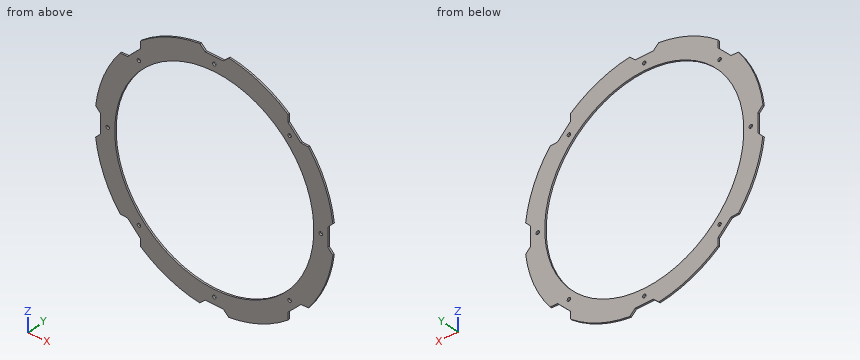
```python
from build123d import *

# Parameters (mm, degrees)
SKETCH1_R           = 3.302
SKETCH1_R_2         = 190.5
BOSS_EXTRUDE1_DEPTH = 3.175
CHAMFER1_DEPTH      = 3.175


with BuildPart() as part:
    # Sketch1 → Boss-Extrude1 (new body)
    with BuildSketch(Plane(origin=(0, 0, 0), x_dir=(1, 0, 0), z_dir=(0, 1, 0))):
        with BuildLine():
            Line((228.003026076, -16.51), (217.17, -16.51))
            Line((217.17, -16.51), (217.17, 16.51))
            Line((217.17, 16.51), (228.003026076, 16.51))
            ThreePointArc((228.003026076, 16.51), (211.198861132, 87.481432639), (172.896818827, 149.548152912))
            Line((172.896818827, 149.548152912), (165.236712628, 141.888046713))
            Line((165.236712628, 141.888046713), (141.888046713, 165.236712628))
            Line((141.888046713, 165.236712628), (149.548152912, 172.896818827))
            ThreePointArc((149.548152912, 172.896818827), (87.481432639, 211.198861132), (16.51, 228.003026076))
            Line((16.51, 228.003026076), (16.51, 217.17))
            Line((16.51, 217.17), (-16.51, 217.17))
            Line((-16.51, 217.17), (-16.51, 228.003026076))
            ThreePointArc((-16.51, 228.003026076), (-87.481432639, 211.198861132), (-149.548152912, 172.896818827))
            Line((-149.548152912, 172.896818827), (-141.888046713, 165.236712628))
            Line((-141.888046713, 165.236712628), (-165.236712628, 141.888046713))
            Line((-165.236712628, 141.888046713), (-172.896818827, 149.548152912))
            ThreePointArc((-172.896818827, 149.548152912), (-211.198861132, 87.481432639), (-228.003026076, 16.51))
            Line((-228.003026076, 16.51), (-217.17, 16.51))
            Line((-217.17, 16.51), (-217.17, -16.51))
            Line((-217.17, -16.51), (-228.003026076, -16.51))
            ThreePointArc((-228.003026076, -16.51), (-211.198861132, -87.481432639), (-172.896818827, -149.548152912))
            Line((-172.896818827, -149.548152912), (-165.236712628, -141.888046713))
            Line((-165.236712628, -141.888046713), (-141.888046713, -165.236712628))
            Line((-141.888046713, -165.236712628), (-149.548152912, -172.896818827))
            ThreePointArc((-149.548152912, -172.896818827), (-87.481432639, -211.198861132), (-16.51, -228.003026076))
            Line((-16.51, -228.003026076), (-16.51, -217.17))
            Line((-16.51, -217.17), (16.51, -217.17))
            Line((16.51, -217.17), (16.51, -228.003026076))
            ThreePointArc((16.51, -228.003026076), (87.481432639, -211.198861132), (149.548152912, -172.896818827))
            Line((149.548152912, -172.896818827), (141.888046713, -165.236712628))
            Line((141.888046713, -165.236712628), (165.236712628, -141.888046713))
            Line((165.236712628, -141.888046713), (172.896818827, -149.548152912))
            ThreePointArc((172.896818827, -149.548152912), (211.198861132, -87.481432639), (228.003026076, -16.51))
        make_face()
        with Locations(Location((-144.133110743, -144.133110743, 0), (0, 0, 270))):
            Circle(SKETCH1_R, mode=Mode.SUBTRACT)
        with Locations(Location((0, -203.835, 0), (0, 0, 270))):
            Circle(SKETCH1_R, mode=Mode.SUBTRACT)
        with Locations(Location((144.133110743, -144.133110743, 0), (0, 0, 270))):
            Circle(SKETCH1_R, mode=Mode.SUBTRACT)
        with Locations(Location((203.835, 0, 0), (0, 0, 270))):
            Circle(SKETCH1_R, mode=Mode.SUBTRACT)
        with Locations(Location((-203.835, 0, 0), (0, 0, 270))):
            Circle(SKETCH1_R, mode=Mode.SUBTRACT)
        with Locations(Location((-144.133110743, 144.133110743, 0), (0, 0, 270))):
            Circle(SKETCH1_R, mode=Mode.SUBTRACT)
        with Locations(Location((0, 0, 0), (0, 0, 270))):
            Circle(SKETCH1_R_2, mode=Mode.SUBTRACT)
        with Locations(Location((0, 203.835, 0), (0, 0, 270))):
            Circle(SKETCH1_R, mode=Mode.SUBTRACT)
        with Locations(Location((144.133110743, 144.133110743, 0), (0, 0, 270))):
            Circle(SKETCH1_R, mode=Mode.SUBTRACT)
    extrude(amount=BOSS_EXTRUDE1_DEPTH)

    # Chamfer1: read off the stored shape, not the designer's step
    # Chamfer1 outline → Chamfer1 (cut)
    with BuildSketch(Plane(origin=(0, 0, 0), x_dir=(1, 0, 0), z_dir=(0, 1, 0))):
        with BuildLine():
            ThreePointArc((228.003026076, 16.51), (227.528537531, 22.1071167), (226.916669439, 27.690885335))
            Line((226.916669439, 27.690885335), (217.17, 17.417305498))
            Line((217.17, 17.417305498), (217.17, 16.51))
            Line((217.17, 16.51), (228.003026076, 16.51))
        make_face()
        with BuildLine():
            Line((165.878274498, 141.246484842), (180.034728522, 140.873902927))
            ThreePointArc((180.034728522, 140.873902927), (176.519063933, 145.254879671), (172.896818827, 149.548152912))
            Line((172.896818827, 149.548152912), (165.236712628, 141.888046713))
            Line((165.236712628, 141.888046713), (165.878274498, 141.246484842))
        make_face()
        with BuildLine():
            Line((228.003026076, -16.51), (217.17, -16.51))
            Line((217.17, -16.51), (217.17, -17.417305498))
            Line((217.17, -17.417305498), (226.916669439, -27.690885335))
            ThreePointArc((226.916669439, -27.690885335), (227.528537531, -22.1071167), (228.003026076, -16.51))
        make_face()
        with BuildLine():
            Line((141.246484842, 165.878274498), (141.888046712, 165.236712627))
            Line((141.888046712, 165.236712627), (149.548152912, 172.896818827))
            ThreePointArc((149.548152912, 172.896818827), (145.254879671, 176.519063933), (140.873902927, 180.034728522))
            Line((140.873902927, 180.034728522), (141.246484842, 165.878274498))
        make_face()
        with BuildLine():
            ThreePointArc((172.896818827, -149.548152912), (176.519063933, -145.254879671), (180.034728522, -140.873902927))
            Line((180.034728522, -140.873902927), (165.878274498, -141.246484842))
            Line((165.878274498, -141.246484842), (165.236712627, -141.888046712))
            Line((165.236712627, -141.888046712), (172.896818827, -149.548152912))
        make_face()
        with BuildLine():
            Line((17.417305498, 217.17), (27.690885335, 226.916669439))
            ThreePointArc((27.690885335, 226.916669439), (22.1071167, 227.528537531), (16.51, 228.003026076))
            Line((16.51, 228.003026076), (16.51, 217.17))
            Line((16.51, 217.17), (17.417305498, 217.17))
        make_face()
        with BuildLine():
            Line((149.548152912, -172.896818827), (141.888046713, -165.236712628))
            Line((141.888046713, -165.236712628), (141.246484842, -165.878274498))
            Line((141.246484842, -165.878274498), (140.873902927, -180.034728522))
            ThreePointArc((140.873902927, -180.034728522), (145.254879671, -176.519063933), (149.548152912, -172.896818827))
        make_face()
        with BuildLine():
            Line((-17.417305498, 217.17), (-16.51, 217.17))
            Line((-16.51, 217.17), (-16.51, 228.003026076))
            ThreePointArc((-16.51, 228.003026076), (-22.1071167, 227.528537531), (-27.690885335, 226.916669439))
            Line((-27.690885335, 226.916669439), (-17.417305498, 217.17))
        make_face()
        with BuildLine():
            ThreePointArc((16.51, -228.003026076), (22.1071167, -227.528537531), (27.690885335, -226.916669439))
            Line((27.690885335, -226.916669439), (17.417305498, -217.17))
            Line((17.417305498, -217.17), (16.51, -217.17))
            Line((16.51, -217.17), (16.51, -228.003026076))
        make_face()
        with BuildLine():
            Line((-141.246484842, 165.878274498), (-140.873902927, 180.034728522))
            ThreePointArc((-140.873902927, 180.034728522), (-145.254879671, 176.519063933), (-149.548152912, 172.896818827))
            Line((-149.548152912, 172.896818827), (-141.888046713, 165.236712628))
            Line((-141.888046713, 165.236712628), (-141.246484842, 165.878274498))
        make_face()
        with BuildLine():
            Line((-16.51, -228.003026076), (-16.51, -217.17))
            Line((-16.51, -217.17), (-17.417305498, -217.17))
            Line((-17.417305498, -217.17), (-27.690885335, -226.916669439))
            ThreePointArc((-27.690885335, -226.916669439), (-22.1071167, -227.528537531), (-16.51, -228.003026076))
        make_face()
        with BuildLine():
            Line((-165.878274498, 141.246484842), (-165.236712627, 141.888046712))
            Line((-165.236712627, 141.888046712), (-172.896818827, 149.548152912))
            ThreePointArc((-172.896818827, 149.548152912), (-176.519063933, 145.254879671), (-180.034728522, 140.873902927))
            Line((-180.034728522, 140.873902927), (-165.878274498, 141.246484842))
        make_face()
        with BuildLine():
            ThreePointArc((-149.548152912, -172.896818827), (-145.254879671, -176.519063933), (-140.873902927, -180.034728522))
            Line((-140.873902927, -180.034728522), (-141.246484842, -165.878274498))
            Line((-141.246484842, -165.878274498), (-141.888046712, -165.236712627))
            Line((-141.888046712, -165.236712627), (-149.548152912, -172.896818827))
        make_face()
        with BuildLine():
            Line((-217.17, 17.417305498), (-226.916669439, 27.690885335))
            ThreePointArc((-226.916669439, 27.690885335), (-227.528537531, 22.1071167), (-228.003026076, 16.51))
            Line((-228.003026076, 16.51), (-217.17, 16.51))
            Line((-217.17, 16.51), (-217.17, 17.417305498))
        make_face()
        with BuildLine():
            Line((-172.896818827, -149.548152912), (-165.236712628, -141.888046713))
            Line((-165.236712628, -141.888046713), (-165.878274498, -141.246484842))
            Line((-165.878274498, -141.246484842), (-180.034728522, -140.873902927))
            ThreePointArc((-180.034728522, -140.873902927), (-176.519063933, -145.254879671), (-172.896818827, -149.548152912))
        make_face()
        with BuildLine():
            Line((-217.17, -17.417305498), (-217.17, -16.51))
            Line((-217.17, -16.51), (-228.003026076, -16.51))
            ThreePointArc((-228.003026076, -16.51), (-227.528537531, -22.1071167), (-226.916669439, -27.690885335))
            Line((-226.916669439, -27.690885335), (-217.17, -17.417305498))
        make_face()
    extrude(amount=CHAMFER1_DEPTH, mode=Mode.SUBTRACT)


solid = part.part
```
CAD build for the part. Positions are in the model's coordinates, mm. Round coordinates to 2 decimals unless told otherwise and drop trailing zeros. Loops run counter-clockwise (first coordinate to the right, second up) from the corner with the lowest first, then second, coordinate; pieces in that order, holes last. Notation, with made-up numbers: M -4.5,51.25 L 6.5,51.25 A18 ccw 6.5,82.25 Z; hole C -40,73.5 d2. An arc over 180 degrees is marked long. Return JSON: item names as keys, results as strings. Group by question number.
(1) Wall check: probe 1 along X at (y, z) = (2.05, 0); probe 2 along Z at (x, y) = (143.5, 0.8); probe 3 along Z at (x, y) = (4, 1.65). Give the ranges that are in metal, low to high. Write a range as [from, to].
(2) Saw through at C-C, the plane y = 0.85. Give the number of separate pieces and of enclosed holes in the cut face, and give its area (3 significant figures).
(3) Saw through at B-B, the plane x = 85. List the corners of the cut face in (y, z) (3 decimals).
(4) Drop flat-ended pins along their axis: P1, Ø1.6, axis at y = 1, z = 0.5, coming from the +X side; P2, Ø1.5, axis at y = 1, z = 72, coming from the -X side; P3, Ø1, axis at x = 0.5, y = 1.5, coming from the -Z side. Give the stop position or say it passes through.
(5) Saw through at A-A, the plane z = -121. List the corners of the cut face in (x, y) (3 decimals), and give its area (3 significant figures).
Answer list:
{
 "1": {"probe 1": "[-217.17, -207.14], [-200.53, -190.5], [190.5, 200.53], [207.14, 217.17]", "probe 2": "[-163.62, -147.37], [-140.89, -125.29], [125.29, 140.89], [147.37, 163.62]", "probe 3": "[-217.17, -190.46], [190.46, 217.17]"},
 "2": {"separate pieces": "1", "enclosed holes": "9", "area": "45,900 mm2"},
 "3": {"outline": "M 0,-212.21 L 3.175,-212.21 L 3.175,-170.485 L 0,-170.485 Z; M 0,170.485 L 3.175,170.485 L 3.175,212.21 L 0,212.21 Z"},
 "4": {"P1": "x = 217.17", "P2": "x = -217.21", "P3": "z = -217.17"},
 "5": {"outline": "M -193.951,0 L -147.137,0 L -147.137,3.175 L -193.951,3.175 Z; M 147.137,0 L 193.951,0 L 193.951,3.175 L 147.137,3.175 Z", "area": "297 mm2"}
}
